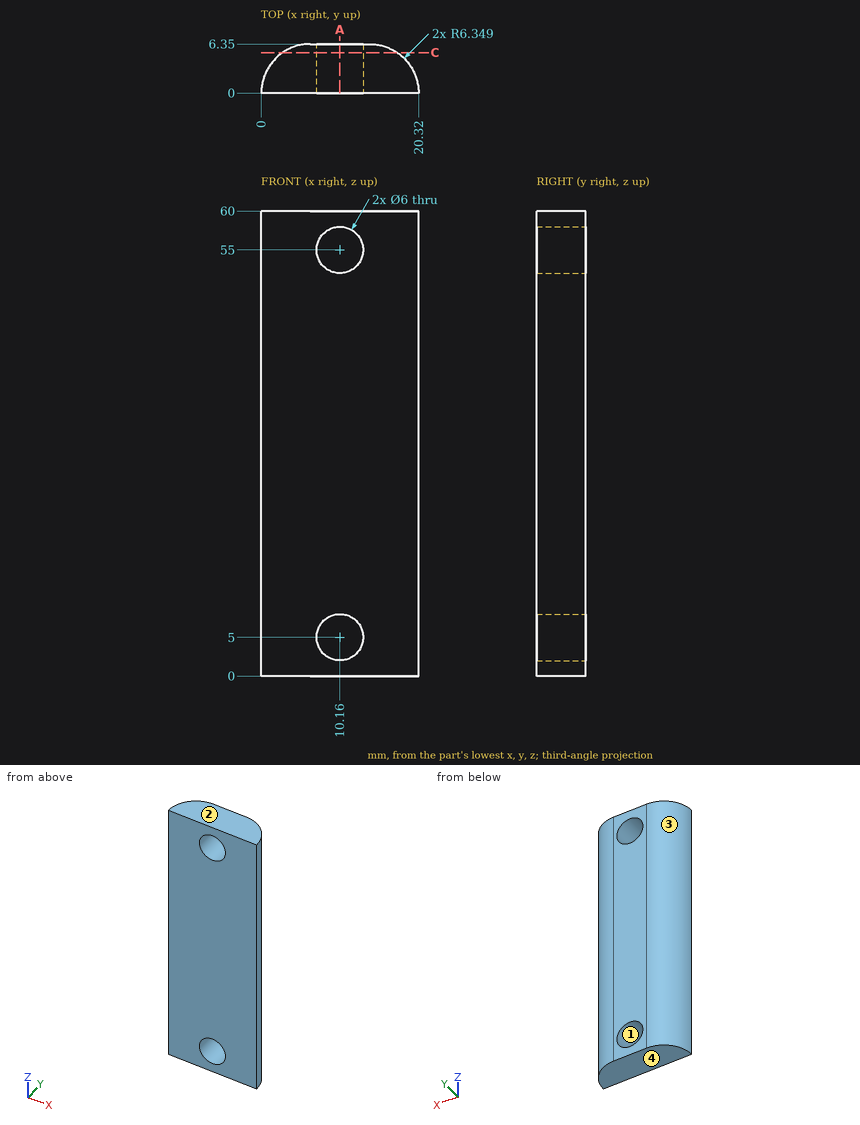
Check sheet for the drawn part. Datum: minimum x, y, z corner. Units: mm. Round coordinates to 2 decimals unless told otherwise and drop trailing zeros. Order: outer loops, then holes, each group sorted by start corner. A loop starts at its lowest first (then second) coordinate and runs counter-clockwise, first axis right, second up.
(1) Go/stop test with flat-tipped pins: P1, Ø3, axis at y = 3.5, z = 27, coming from the +X side; P2, Ø3, axis at y = 2, z = 14, coming from the +X side; P3, Ø5, axis at x = 10.16, z = 5, coming from the +Y side. Record where each tip stops, or that it passes through.
(2) Cross-section at A-A, the plane x = 10.16. Enter the section's corners in (y, z).
(3) Draft check along Z on the marked faces 1, 2, 3 and 4. Enter one of: pulls with the +Z half, pulls with the -Z half, needs draft (parallel to the pull), parting line crosses it, or undercut.
(4) Scan lines: probe 1 along Z at (x, y) = (10.25, 5); probe 2 along Z at (x, y) = (11, 4.75); probe 3 along Y at (x, z) = (6, 49.5). Record each from-to range of solid material in increasing order.
(5) Cross-section at C-C, the plane y = 5.25. Enter the section's corners in (x, z).
Check sheet entries:
1. P1: stops at x = 20
1. P2: stops at x = 20.3
1. P3: passes through
2. outline: (0, 0) - (6.35, 0) - (6.35, 2) - (0, 2) - close; (0, 8) - (6.35, 8) - (6.35, 52) - (0, 52) - close; (0, 58) - (6.35, 58) - (6.35, 60) - (0, 60) - close
3. face 1: undercut
3. face 2: pulls with the +Z half
3. face 3: needs draft
3. face 4: pulls with the -Z half
4. probe 1: z = 0 to 2, 8 to 52, 58 to 60
4. probe 2: z = 0 to 2.12, 7.88 to 52.12, 57.88 to 60
4. probe 3: y = 0 to 6.34
5. outline: (2.78, 0) - (17.54, 0) - (17.54, 60) - (2.78, 60) - close; hole circle Ø6 at (10.16, 5); hole circle Ø6 at (10.16, 55)
